Input: part model. Units: mm. Frame: model coordinates. Face numbers are marked on the shaded views. A direction names the side the tool comes from. Give positions to 0.01 mm unless a question says otherwise; leave off trailing zeros. Loops run counter-clockwise (first coordinate to the right, second up) from the corner with the lowest first, then second, coordinate; pieces in that order, holes last. Notation, with made-up numbers: (39, 13.5) -> (44, 13.5) arc R34 ccw to (44, 43.5) -> close; hole circle Ø6 at (71, 49.25). An arc over 180 degrees is marked (long way). Answer in a Markdown table with one row per item. Add a question column.
```python
from build123d import *

# Parameters (mm, degrees)
SKETCH_1_R                   = 16
EXTRUDE_1_DEPTH              = 8
HOLE_WIZARD_M4_1_D           = 3.3
HOLE_WIZARD_M4_1_DEPTH       = 6
HOLE_WIZARD_M4_1_CSINK_D     = 4.05
HOLE_WIZARD_M4_1_CSINK_ANGLE = 90
HOLE_WIZARD_M4_1_TIP         = 0.991420021
SKETCH_5_R                   = 2
CUT_EXTRUDE_1_DEPTH          = 8
SKETCH_6_R                   = 5
CUT_EXTRUDE_2_DEPTH          = 8


with BuildPart() as part:
    # 草图1 → 凸台-拉伸1 (new body)
    with BuildSketch(Plane(origin=(0, 0, 0), x_dir=(1, 0, 0), z_dir=(0, 1, 0))):
        with Locations(Location((0, 0, 0), (0, 0, 270))):
            Circle(SKETCH_1_R)
    extrude(amount=EXTRUDE_1_DEPTH)

    # M4 螺纹孔1
    with Locations(Plane(origin=(0, 8, 0), x_dir=(1, 0, 0), z_dir=(0, 1, 0))):
        with Locations((-11.400524182, 3.745403632), (-2.456647399, 11.745845374), (8.943876784, 8.000441742), (11.400524182, -3.745403632), (2.456647399, -11.745845374), (-8.943876784, -8.000441742)):
            CounterSinkHole(HOLE_WIZARD_M4_1_D / 2, HOLE_WIZARD_M4_1_CSINK_D / 2, depth=HOLE_WIZARD_M4_1_DEPTH, counter_sink_angle=HOLE_WIZARD_M4_1_CSINK_ANGLE)
            with Locations((0, 0, -(HOLE_WIZARD_M4_1_DEPTH + HOLE_WIZARD_M4_1_TIP / 2))):  # 118° drill point
                Cone(0, HOLE_WIZARD_M4_1_D / 2, HOLE_WIZARD_M4_1_TIP, mode=Mode.SUBTRACT)

    # 草图5 → 切除-拉伸1 (cut)
    with BuildSketch(Plane(origin=(0, 8, 0), x_dir=(1, 0, 0), z_dir=(0, 1, 0))):
        with Locations(Location((3.646912878, 11.432411227, 0), (0, 0, 270))):
            Circle(SKETCH_5_R)
        with Locations(Location((8.07730211, -8.874524811, 0), (0, 0, 270))):
            Circle(SKETCH_5_R)
        with Locations(Location((-11.724214988, -2.557886415, 0), (0, 0, 270))):
            Circle(SKETCH_5_R)
    extrude(amount=-CUT_EXTRUDE_1_DEPTH, mode=Mode.SUBTRACT)

    # 草图6 → 切除-拉伸2 (cut)
    with BuildSketch(Plane(origin=(0, 8, 0), x_dir=(1, 0, 0), z_dir=(0, 1, 0))):
        with Locations(Location((0, 0, 0), (0, 0, 270))):
            Circle(SKETCH_6_R)
    extrude(amount=-CUT_EXTRUDE_2_DEPTH, mode=Mode.SUBTRACT)


solid = part.part
```
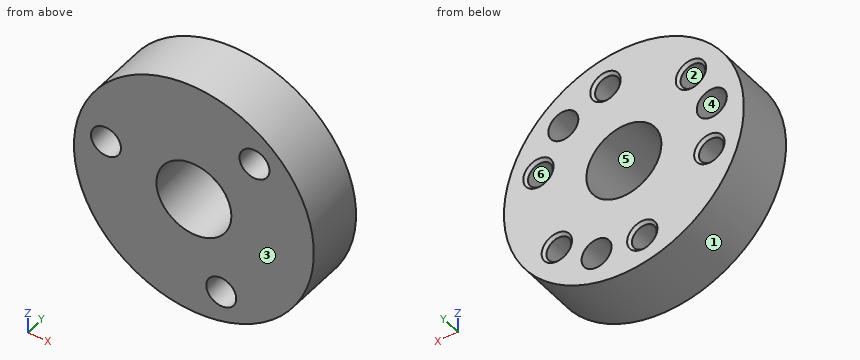
1) Material intervals for line 1 along X through (y, z) = (2, 0); line 2 along X through (y, z) = (7.25, 9); line 3 along X through (y, z) = (5.5, 2), sorted ascending.
2) Pull-direction query (X, two-part tool) for the marked faces 1, 2, 3 and 4; classes: +X half, -X half, draft (parallel to the pull), parting line (faces both ways), or undercut.
3) Section C-C on y = 4.5. State how many separate pieces and enclosed holes the cut face has, and give its area (3 significant figures).
4) Section D-D on z = 14.5. Output: boundary loops of the cut face in (x, y), and give its area (3 significant figures).
5) Section B-B on z = 0. Output: boundary loops of the cut face in (x, y), and give its area (3 significant figures).
6) Reachability of the marked faces 5 and 6 from +Z, -Z, +X, -X, +Y, -Y: full face, straight path, thin tool, end or side. Return the list, or none.
7) Pin query (flat end, axial travel): pin 1 (3 mm diameter, centred on x = 11.4, z = 3.75, fed in from +Y); pin 2 (2 mm diameter, centred on x = 0, z = -3, fed in from -Y); pin 3 (4 mm diameter, centred on y = 6.5, z = -2.5, fed in from -X); pin 4 (1.5 mm diameter, centred on y = 2.5, z = 8.5, fed in from +X). Return the tip coordinate at first contact, or that it passes through.
8) Section A-A on x = 0. Output: boundary loops of the cut face in (y, z).
Working result:
| question | item | result |
|---|---|---|
| 1 | line 1 | x = -16 to -5, 5 to 16 |
| 1 | line 2 | x = -13.23 to -10.26, -7.63 to 6.08, 10.07 to 13.23 |
| 1 | line 3 | x = -15.87 to -13.64, -9.8 to -4.58, 4.58 to 15.87 |
| 2 | face 1 | parting line |
| 2 | face 2 | undercut |
| 2 | face 3 | draft |
| 2 | face 4 | undercut |
| 3 | separate pieces | 1 |
| 3 | enclosed holes | 10 |
| 3 | area | 637 mm2 |
| 4 | outline | (-6.76, 0) -> (6.76, 0) -> (6.76, 8) -> (-6.76, 8) -> close |
| 4 | area | 108 mm2 |
| 5 | outline | (-16, 0) -> (-5, 0) -> (-5, 8) -> (-16, 8) -> close; (5, 0) -> (16, 0) -> (16, 8) -> (5, 8) -> close |
| 5 | area | 176 mm2 |
| 6 | face 5 | +Y, -Y |
| 6 | face 6 | +Y |
| 7 | pin 1 | stops at y = 1.91 |
| 7 | pin 2 | passes through |
| 7 | pin 3 | stops at x = -15.99 |
| 7 | pin 4 | stops at x = 14 |
| 8 | outline | (0, -16) -> (8, -16) -> (8, -5) -> (0, -5) -> close; (0, 5) -> (8, 5) -> (8, 16) -> (0, 16) -> close |
